from build123d import *

# Parameters (mm, degrees)
EXTRUDE_THIN1_DEPTH                   = 137.50025
EXTRUDE_THIN1_DEPTH_BACK              = 213.5
BOSS_EXTRUDE1_DEPTH                   = 212.50025
BOSS_EXTRUDE1_DEPTH_BACK              = 288.5
SKETCH3_OUTSIDE_W                     = 604.22
SKETCH3_OUTSIDE_H                     = 158.409
SKETCH3_OUTSIDE_W_2                   = 500
SKETCH3_OUTSIDE_H_2                   = 100
CUT_EXTRUDE1_DEPTH                    = 47.9721863
F_1_4_20_TAPPED_HOLE1_D               = 5.1054
F_1_4_20_TAPPED_HOLE1_DEPTH           = 16.51
F_1_4_20_TAPPED_HOLE1_TIP             = 1.533816902
F_1_4_20_TAPPED_HOLE1_ON_FACE_2_D     = 5.1054
F_1_4_20_TAPPED_HOLE1_ON_FACE_2_DEPTH = 16.51
F_1_4_20_TAPPED_HOLE1_ON_FACE_2_TIP   = 1.533816902


with BuildPart() as part:
    # Sketch1 → Extrude-Thin1 (new body, two sides)
    with BuildSketch(Plane.XY) as extrude_thin1_sk:
        with BuildLine():
            Line((-1, 27.377741566), (-1, 77.801426032))
            ThreePointArc((-1, 77.801426032), (-1.350622843, 78.765237295), (-2.238576202, 79.278469565))
            Line((-2.238576202, 79.278469565), (-14.558703221, 81.459024387))
            ThreePointArc((-14.558703221, 81.459024387), (-15.894736771, 81.028505523), (-16.289731152, 79.681541685))
            Line((-16.289731152, 79.681541685), (-16.133756174, 78.918587001))
            ThreePointArc((-16.133756174, 78.918587001), (-16.425245763, 77.689683441), (-17.551976749, 77.11902818))
            Line((-17.551976749, 77.11902818), (-31.176844118, 76.65202466))
            ThreePointArc((-31.176844118, 76.65202466), (-32.394172225, 75.953136671), (-32.500485501, 74.553483275))
            Line((-32.500485501, 74.553483275), (-32.189291753, 73.839630003))
            ThreePointArc((-32.189291753, 73.839630003), (-32.218908178, 72.576976841), (-33.202371488, 71.784531222))
            Line((-33.202371488, 71.784531222), (-46.048094302, 68.590520723))
            ThreePointArc((-46.048094302, 68.590520723), (-47.095522714, 67.648327859), (-46.899674588, 66.253165796))
            Line((-46.899674588, 66.253165796), (-18.735090298, 27.487941181))
            ThreePointArc((-18.735090298, 27.487941181), (-17.958226336, 26.809018221), (-16.963801619, 26.534111898))
            Line((-16.963801619, 26.534111898), (-2.568160686, 25.879290992))
            ThreePointArc((-2.568160686, 25.879290992), (-1.463718433, 26.293250665), (-1, 27.377741566))
        make_face()
        with BuildLine():
            Line((-1.27, 27.377741566), (-1.27, 77.801426032))
            ThreePointArc((-1.27, 77.801426032), (-1.557510731, 78.591751268), (-2.285632486, 79.012601729))
            Line((-2.285632486, 79.012601729), (-14.605759505, 81.193156552))
            ThreePointArc((-14.605759505, 81.193156552), (-15.701307016, 80.840131082), (-16.025202408, 79.735620736))
            Line((-16.025202408, 79.735620736), (-15.86922743, 78.972666052))
            ThreePointArc((-15.86922743, 78.972666052), (-16.213185146, 77.522559851), (-17.542727708, 76.849186643))
            Line((-17.542727708, 76.849186643), (-31.167595078, 76.382183123))
            ThreePointArc((-31.167595078, 76.382183123), (-32.165804125, 75.809094972), (-32.252981012, 74.661379187))
            Line((-32.252981012, 74.661379187), (-31.941787264, 73.947525915))
            ThreePointArc((-31.941787264, 73.947525915), (-31.976734646, 72.457595184), (-33.137221351, 71.522509354))
            Line((-33.137221351, 71.522509354), (-45.982944165, 68.328498854))
            ThreePointArc((-45.982944165, 68.328498854), (-46.841835463, 67.555900706), (-46.68124, 66.411867814))
            Line((-46.68124, 66.411867814), (-18.516655709, 27.646643199))
            ThreePointArc((-18.516655709, 27.646643199), (-17.830213301, 27.046742143), (-16.951532696, 26.803833001))
            Line((-16.951532696, 26.803833001), (-2.555891763, 26.149012095))
            ThreePointArc((-2.555891763, 26.149012095), (-1.650249115, 26.488459027), (-1.27, 27.377741566))
        make_face(mode=Mode.SUBTRACT)
    extrude(amount=EXTRUDE_THIN1_DEPTH)
    extrude(extrude_thin1_sk.sketch, amount=-EXTRUDE_THIN1_DEPTH_BACK)


with BuildPart() as body_2:
    # Sketch2 → Boss-Extrude1 (new body, two sides)
    with BuildSketch(Plane.XY) as boss_extrude1_sk:
        with BuildLine():
            Line((-46.68124, 66.411867814), (-18.516655709, 27.646643199))
            ThreePointArc((-18.516655709, 27.646643199), (-17.830213301, 27.046742143), (-16.951532696, 26.803833001))
            Line((-16.951532696, 26.803833001), (-2.555891763, 26.149012095))
            ThreePointArc((-2.555891763, 26.149012095), (-1.650249115, 26.488459027), (-1.27, 27.377741566))
            Line((-1.27, 27.377741566), (-1.27, 77.801426032))
            Line((-1.27, 77.801426032), (-1.27, 77.950492711))
            ThreePointArc((-1.27, 77.950492711), (-1.551343626, 78.723865471), (-2.263847169, 79.13568869))
            Line((-2.263847169, 79.13568869), (-14.583974188, 81.316243513))
            ThreePointArc((-14.583974188, 81.316243513), (-15.790857829, 80.927341471), (-16.147669419, 79.710584138))
            Line((-16.147669419, 79.710584138), (-15.991694441, 78.947629454))
            ThreePointArc((-15.991694441, 78.947629454), (-16.311361358, 77.599931884), (-17.547009672, 76.97411328))
            Line((-17.547009672, 76.97411328), (-31.171877041, 76.50710976))
            ThreePointArc((-31.171877041, 76.50710976), (-32.271530097, 75.875780943), (-32.367566424, 74.611427376))
            Line((-32.367566424, 74.611427376), (-32.056372675, 73.897574104))
            ThreePointArc((-32.056372675, 73.897574104), (-32.088852022, 72.51286447), (-33.167383452, 71.643815774))
            Line((-33.167383452, 71.643815774), (-46.013106265, 68.449805275))
            ThreePointArc((-46.013106265, 68.449805275), (-46.895812161, 67.655785191), (-46.730763846, 66.48003154))
            Line((-46.730763846, 66.48003154), (-46.68124, 66.411867814))
        make_face()
    extrude(amount=BOSS_EXTRUDE1_DEPTH)
    extrude(boss_extrude1_sk.sketch, amount=-BOSS_EXTRUDE1_DEPTH_BACK)

    # Sketch3 outside → Cut-Extrude1 (cut, through all)
    with BuildSketch(Plane(origin=(0, 0, 0), x_dir=(0, 0, -1), z_dir=(1, 0, 0))):
        with Locations((38, 53.7425)):
            Rectangle(SKETCH3_OUTSIDE_W, SKETCH3_OUTSIDE_H)
        with Locations((37.999875, 52.664117138)):
            Rectangle(SKETCH3_OUTSIDE_W_2, SKETCH3_OUTSIDE_H_2, mode=Mode.SUBTRACT)
    extrude(amount=-CUT_EXTRUDE1_DEPTH, mode=Mode.SUBTRACT)

    # 1/4-20 Tapped Hole1
    with Locations(Plane(origin=(-13.27, 65.164117138, 212.000125), x_dir=(1, 0, 0), z_dir=(0, 0, 1))):
        with Locations((0, 0), (0, -25)):
            Hole(F_1_4_20_TAPPED_HOLE1_D / 2, depth=F_1_4_20_TAPPED_HOLE1_DEPTH)
            with Locations((0, 0, -(F_1_4_20_TAPPED_HOLE1_DEPTH + F_1_4_20_TAPPED_HOLE1_TIP / 2))):  # 118° drill point
                Cone(0, F_1_4_20_TAPPED_HOLE1_D / 2, F_1_4_20_TAPPED_HOLE1_TIP, mode=Mode.SUBTRACT)

    # 1/4-20 Tapped Hole1 on face 2
    with Locations(Plane(origin=(-13.27, 65.164117138, -287.999875), x_dir=(-1, 0, 0), z_dir=(0, 0, -1))):
        with Locations((0, 0), (0, -25)):
            Hole(F_1_4_20_TAPPED_HOLE1_ON_FACE_2_D / 2, depth=F_1_4_20_TAPPED_HOLE1_ON_FACE_2_DEPTH)
            with Locations((0, 0, -(F_1_4_20_TAPPED_HOLE1_ON_FACE_2_DEPTH + F_1_4_20_TAPPED_HOLE1_ON_FACE_2_TIP / 2))):  # 118° drill point
                Cone(0, F_1_4_20_TAPPED_HOLE1_ON_FACE_2_D / 2, F_1_4_20_TAPPED_HOLE1_ON_FACE_2_TIP, mode=Mode.SUBTRACT)


solid = body_2.part
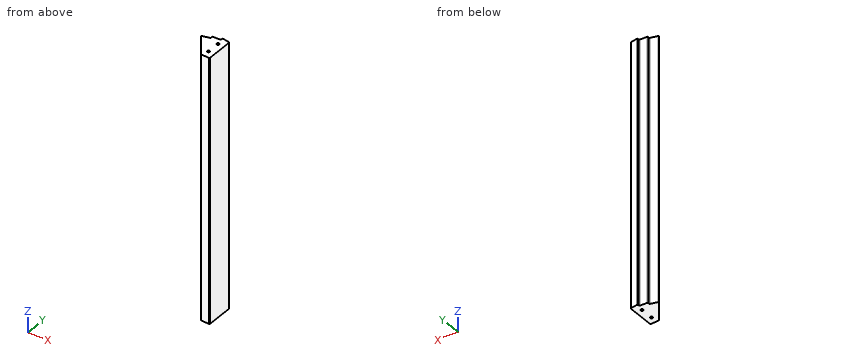
The model under review builds one solid part; all positions refer to its coordinate system, in mm. Round coordinates to 2 decimals unless told otherwise and drop trailing zeros. Loops run counter-clockwise (first coordinate to the right, second up) from the corner with the lowest first, then second, coordinate; pieces in that order, holes last. Notation, with made-up numbers: M 35,-20.5 L 82,-20.5 A20 cw 82,12.5 Z; hole C -37.75,-14.5 d11. An arc over 180 degrees is marked long. Answer as a JSON object with one key per item and string values.
Item 1: Clearance check with flat-ended pins moving along their axes: P1, Ø1.5, axis at x = -11, z = -31, coming from the +Y side; P2, Ø5, axis at x = -24, z = -80.5, coming from the -Y side; P3, Ø10, axis at x = -9, z = -9, coming from the +Y side. State where each tip first meets the part, or that it passes through.
Check sheet entries:
{"P1": "y = 80.81", "P2": "y = 31.75", "P3": "y = 81.21"}
Item 2: We need section A-A, the plane z = 9.5. State the section outline as (x, y) points (1 decimal), and give its area (3 significant figures).
Check sheet entries:
{"outline": "M -46.7,66.5 L -18.5,27.6 A2 ccw -17,26.8 L -2.6,26.1 A1.2 ccw -1.3,27.4 L -1.3,78 A1.2 ccw -2.3,79.1 L -14.6,81.3 A1.4 ccw -16.1,79.7 L -16,78.9 A1.6 cw -17.5,77 L -31.2,76.5 A1.4 ccw -32.4,74.6 L -32.1,73.9 A1.6 cw -33.2,71.6 L -46,68.4 A1.3 ccw Z", "area": "1,660 mm2"}
Item 3: For line 1 along Y through (x, z) = (-13, -278); line 2 along Y through (x, z) = (-13.27, -275.5); line 3 along X through (y, z) = (72, 58), list the stretches that pass through material, from the lowest coordinate up.
Check sheet entries:
{"line 1": "26.62 to 37.63, 42.7 to 62.63, 67.7 to 81.04", "line 2": "26.64 to 37.61, 42.72 to 62.61, 67.72 to 81.08", "line 3": "-32.48 to -1.27"}
